The listing builds one solid part. Answer for the finished solid, in the listing's coordinates (mm). A direction names the side the tool comes from. Round coordinates to 2 decimals unless told otherwise and drop trailing zeros. Write each loop counter-clockwise with the first axis right and the second up, starting at its lowest first coordinate (ties: lowest second). Pieces come first, ordered by that corner, then holes.
from build123d import *

# Parameters (mm, degrees)
BOSS_EXTRUDE1_DEPTH     = 20
CUT_EXTRUDE_THIN1_DEPTH = 17
FILLET1_R               = 10
SKETCH3_R               = 3.75
SKETCH3_R_2             = 2.25
CUT_EXTRUDE1_DEPTH      = 17
SKETCH3_2_R             = 2.25
CUT_EXTRUDE2_DEPTH      = 207.700266086
FILLET2_R               = 3
SKETCH4_W               = 5
SKETCH4_H               = 5.1
CUT_EXTRUDE3_DEPTH      = 207.43158673


with BuildPart() as part:
    # Sketch1 → Boss-Extrude1 (new body)
    with BuildSketch(Plane.XY):
        Polygon((-115, 0), (-175.5, 0), (-175.5, 80.5), (175.5, 80.5), (175.5, 0), (115, 0), (115, -9.5), (185, -9.5), (185, 90), (-185, 90), (-185, -9.5), (-115, -9.5), align=None)
    extrude(amount=BOSS_EXTRUDE1_DEPTH)

    # Sketch2 → Cut-Extrude-Thin1 (cut)
    with BuildSketch(Plane.XY.offset(20)):
        Polygon((-125, -2.2), (-177.7, -2.2), (-177.7, 82.7), (177.7, 82.7), (177.7, -2.2), (125, -2.2), (125, -7.3), (182.8, -7.3), (182.8, 87.8), (-182.8, 87.8), (-182.8, -7.3), (-125, -7.3), align=None)
    extrude(amount=-CUT_EXTRUDE_THIN1_DEPTH, mode=Mode.SUBTRACT)

    # Fillet1
    fillet1_edges = [part.edges().sort_by_distance(p)[0] for p in [
        (175.5, 0, 10),
        (175.5, 80.5, 10),
        (-175.5, 80.5, 10),
        (-175.5, 0, 10),
        (-177.7, -2.2, 11.5),
        (-177.7, 82.7, 11.5),
        (177.7, 82.7, 11.5),
        (177.7, -2.2, 11.5),
    ]]
    fillet(fillet1_edges, radius=FILLET1_R)

    # Sketch3 → Cut-Extrude1 (cut)
    # profile 1 of 4: a face of its own
    with BuildSketch(Plane.XY.offset(20)):
        with Locations((-120, 85.25)):
            Circle(SKETCH3_R)
        with Locations((-120, 85.25)):
            Circle(SKETCH3_R_2, mode=Mode.SUBTRACT)
    # profile 2 of 4: a face of its own
    with BuildSketch(Plane.XY.offset(20)):
        with Locations((120, 85.25)):
            Circle(SKETCH3_R)
        with Locations((120, 85.25)):
            Circle(SKETCH3_R_2, mode=Mode.SUBTRACT)
    # profile 3 of 4: a face of its own
    with BuildSketch(Plane.XY.offset(20)):
        with Locations((-155, -4.75)):
            Circle(SKETCH3_R)
        with Locations((-155, -4.75)):
            Circle(SKETCH3_R_2, mode=Mode.SUBTRACT)
    # profile 4 of 4: a face of its own
    with BuildSketch(Plane.XY.offset(20)):
        with Locations((155, -4.75)):
            Circle(SKETCH3_R)
        with Locations((155, -4.75)):
            Circle(SKETCH3_R_2, mode=Mode.SUBTRACT)
    extrude(amount=-CUT_EXTRUDE1_DEPTH, mode=Mode.SUBTRACT)

    # Sketch3<2> → Cut-Extrude2 (cut, through all)
    with BuildSketch(Plane.XY.offset(20)):
        with Locations((-120, 85.25)):
            Circle(SKETCH3_2_R)
        with Locations((-155, -4.75)):
            Circle(SKETCH3_2_R)
        with Locations((155, -4.75)):
            Circle(SKETCH3_2_R)
        with Locations((120, 85.25)):
            Circle(SKETCH3_2_R)
    extrude(amount=-CUT_EXTRUDE2_DEPTH, mode=Mode.SUBTRACT)

    # Fillet2
    fillet2_edges = [part.edges().sort_by_distance(p)[0] for p in [
        (-115, -9.5, 10),
        (-185, -9.5, 10),
        (-185, 90, 10),
        (185, 90, 10),
        (185, -9.5, 10),
        (115, -9.5, 10),
        (115, 0, 10),
        (-115, 0, 10),
    ]]
    fillet(fillet2_edges, radius=FILLET2_R)

    # Sketch4 → Cut-Extrude3 (cut, through all)
    with BuildSketch(Plane.XY.offset(3)):
        with Locations((-127.5, -4.75)):
            Rectangle(SKETCH4_W, SKETCH4_H)
        with Locations((127.5, -4.75)):
            Rectangle(SKETCH4_W, SKETCH4_H)
    extrude(amount=-CUT_EXTRUDE3_DEPTH, mode=Mode.SUBTRACT)


solid = part.part
1. Section B-B on y = 66 is taken. Determine the outline of the cut face in (x, z), plus the area to 3 significant figures.
Geometry says:
outline: (-185, 0) - (-175.5, 0) - (-175.5, 20) - (-177.7, 20) - (-177.7, 3) - (-182.8, 3) - (-182.8, 20) - (-185, 20) - close; (175.5, 0) - (185, 0) - (185, 20) - (182.8, 20) - (182.8, 3) - (177.7, 3) - (177.7, 20) - (175.5, 20) - close
area: 207 mm2
2. Straight lines are drawn through the part: line 1 along Y through (x, z) = (-155, 1.1); line 2 along Y through (x, z) = (-120, 2.15); line 3 along X through (y, z) = (14.5, 16.5). For each, find the intervals that lie inside material, in ascending order.
Geometry says:
line 1: y = -9.5 to -7, -2.5 to 0, 80.5 to 90
line 2: y = -9.5 to 0, 80.5 to 83, 87.5 to 90
line 3: x = -185 to -182.8, -177.7 to -175.5, 175.5 to 177.7, 182.8 to 185
3. Section A-A on x = -133.5 is taken. Determine the outline of the cut face in (y, z).
Geometry says:
outline: (-9.5, 0) - (0, 0) - (0, 20) - (-2.2, 20) - (-2.2, 3) - (-7.3, 3) - (-7.3, 20) - (-9.5, 20) - close; (80.5, 0) - (90, 0) - (90, 20) - (87.8, 20) - (87.8, 3) - (82.7, 3) - (82.7, 20) - (80.5, 20) - close
4. Section C-C on x = -16 is taken. Determine the outline of the cut face in (y, z).
Geometry says:
outline: (80.5, 0) - (90, 0) - (90, 20) - (87.8, 20) - (87.8, 3) - (82.7, 3) - (82.7, 20) - (80.5, 20) - close
5. Given pin 1 (1.5 mm diameter, centred on x = 23, z = 11.5, fed in from -Y); pin 2 (7 mm diameter, centred on x = -120, y = 85.25, fed in from +Z), each flat-ended and moving along its own axis, determine where each tip first touches the part or whether it passes through.
Geometry says:
pin 1: stops at y = 80.5
pin 2: stops at z = 3
6. A tool of negligible diameter and unlimited length cuts with its end or side. For faces 1 (the face through (174.69, 79.85, 11.38)), 2 (the face through (-150, -9.5, 10)), 3 (the face through (-2, 80.5, 10)), from which of +Z, -Z, +X, -X, +Y, -Y can it reach the whole face along a straight path? Write none if from no direction.
Geometry says:
face 1: +Z
face 2: +Z, -Z, +X, -X, -Y
face 3: +Z, -Z
